from build123d import *

# Parameters (mm, degrees)
F_01_START                             = -3
S01_SOCKET_HEAD_R                      = 3.5
F_01_SOCKET_HEAD_DEPTH                 = 3
S02_GROUND_SHOULDER_R                  = 2
F_02_GROUND_SHOULDER_DEPTH             = 10
F_03_START                             = 10
S03_THREADED_TIP_MAJOR_DIAMETER_R      = 1.5
F_03_THREADED_TIP_MAJOR_DIAMETER_DEPTH = 7
F_04_START                             = -3.1
F_04_HEXAGONAL_DRIVE_DEPTH             = 2.14


with BuildPart() as part:
    # S01 - Socket head → 01 - Socket head (new body)
    with BuildSketch(Plane.XY.offset(F_01_START)):
        Circle(S01_SOCKET_HEAD_R)
    extrude(amount=F_01_SOCKET_HEAD_DEPTH)

    # S02 - Ground shoulder → 02 - Ground shoulder (add)
    with BuildSketch(Plane.XY):
        Circle(S02_GROUND_SHOULDER_R)
    extrude(amount=F_02_GROUND_SHOULDER_DEPTH)

    # S03 - Threaded tip major diameter → 03 - Threaded tip major diameter (add)
    with BuildSketch(Plane.XY.offset(F_03_START)):
        Circle(S03_THREADED_TIP_MAJOR_DIAMETER_R)
    extrude(amount=F_03_THREADED_TIP_MAJOR_DIAMETER_DEPTH)

    # S04 - Hexagonal drive → 04 - Hexagonal drive (cut)
    with BuildSketch(Plane.XY.offset(F_04_START)):
        Polygon((1.154700538, 0), (0.577350269, 1), (-0.577350269, 1), (-1.154700538, 0), (-0.577350269, -1), (0.577350269, -1), align=None)
    extrude(amount=F_04_HEXAGONAL_DRIVE_DEPTH, mode=Mode.SUBTRACT)


solid = part.part
CAD build for the part. Positions are in the model's coordinates, mm. A direction names the side the tool comes from. Round coordinates to 2 decimals unless told otherwise and drop trailing zeros. Loops run counter-clockwise (first coordinate to the right, second up) from the corner with the lowest first, then second, coordinate; pieces in that order, holes last.
(1) Two-plate mould, pull along X, no slides. Class faces 4 (the flat face through (0, 0, 17)), 5 (the cylindrical face through (3.233, -1.341, -1.521)), 6 (the flat face through (0, 0, -0.96)): +X half, -X half, draft (parallel to the pull), parting line (faces both ways), or undercut.
(2) Wall check: line 1 along Z through (x, y) = (2.5, 1.5); line 2 along Z through (x, y) = (-1.5, -0.75); line 3 along Y through (x, z) = (-0.75, -1.5). Give the ranges that are in metal, low to high.
(3) Cut at B-B (z = 11.25). Give the cut face in (x, y).
(4) Cut at A-A (x = 0). Give the cut face in (y, z), plus the area to 3 significant figures.
(5) Drop flat-ended pins along their axis: pin 1 (1.5 mm diameter, centred on y = -2.5, z = 2, fed in from -X); pin 2 (3 mm diameter, centred on x = 0.5, z = 6.5, fed in from +Y); pin 3 (1.5 mm diameter, centred on x = 1.5, y = 0.5, fed in from +Z); pin 4 (1 mm diameter, centred on x = 0, y = 0, fed in from -Z). Give the stop position or say it passes through.
(6) Cut at C-C (y = 2.75). Give the cut face in (x, z).
(7) Which spindle directions (+Z, -Z, +X, -X, +Y, -Y) get a long thin tool onto all of the face, cutting with end or side? Do faces 1 (the flat face through (1, 1, -3)), 2 (the flat face through (2, -2, 0)), 3 (the flat face through (-0.86, 0.51, -1.99)). Say none if no direction does.
(8) Cut at D-D (z = 1.25). Give the cut face in (x, y), plus the area to 3 significant figures.
Findings below:
1. face 4: draft
1. face 5: parting line
1. face 6: undercut
2. line 1: z = -3 to 0
2. line 2: z = -3 to 10
2. line 3: y = -3.42 to -0.7, 0.7 to 3.42
3. outline: circle Ø3 at (0, 0)
4. outline: (-3.5, -3) - (-1, -3) - (-1, -0.96) - (1, -0.96) - (1, -3) - (3.5, -3) - (3.5, 0) - (2, 0) - (2, 10) - (1.5, 10) - (1.5, 17) - (-1.5, 17) - (-1.5, 10) - (-2, 10) - (-2, 0) - (-3.5, 0) - close
4. area: 77.9 mm2
5. pin 1: stops at x = -0.97
5. pin 2: stops at y = 2
5. pin 3: stops at z = 17
5. pin 4: stops at z = -0.96
6. outline: (-2.17, -3) - (2.17, -3) - (2.17, 0) - (-2.17, 0) - close
7. face 1: -Z, +X, -X, +Y, -Y
7. face 2: +Z
7. face 3: -Z
8. outline: circle Ø4 at (0, 0)
8. area: 12.6 mm2
